The listing builds one solid part. Answer for the finished solid, in the listing's coordinates (mm). Coordinates: 2 decimals unless noted, no trailing zeros. Write each loop counter-clockwise with the first axis right and the second up, starting at its lowest first coordinate (ties: lowest second). Pieces come first, ordered by that corner, then holes. Notation, with made-up numbers: M 62,-19 L 93,-19 A24 ccw 93,-9 Z; hole C 44,19.5 d1. An arc over 180 degrees is marked long. Answer as CSV lines item,"result".
```python
from build123d import *

# Parameters (mm, degrees)
SKETCH_1_R      = 3.127436884
SKETCH_1_R_2    = 2.290236854
SKETCH_1_R_3    = 3.334332824
SKETCH_1_R_4    = 3
SKETCH_1_R_5    = 1.883976709
SKETCH_1_R_6    = 2.353930843
SKETCH_1_R_7    = 1.55
EXTRUDE_1_DEPTH = 1.5


with BuildPart() as part:
    # 草图1 → 凸台-拉伸1 (new body)
    with BuildSketch(Plane(origin=(0, 0, 0), x_dir=(1, 0, 0), z_dir=(0, 1, 0))):
        Polygon((-30, 10), (-30, 0), (0, 0), (30, 0), (30, 10), align=None)
        with Locations((17.823374051, 5.840236854)):
            Circle(SKETCH_1_R, mode=Mode.SUBTRACT)
        with Locations((12.171443923, 3.55)):
            Circle(SKETCH_1_R_2, mode=Mode.SUBTRACT)
        with Locations((4.963185209, 5.738422027)):
            Circle(SKETCH_1_R_3, mode=Mode.SUBTRACT)
        with Locations((-4.210962245, 6.229894212)):
            Circle(SKETCH_1_R_4, mode=Mode.SUBTRACT)
        with Locations((-12.074517206, 2.707676886)):
            Circle(SKETCH_1_R_5, mode=Mode.SUBTRACT)
        with Locations((-17.808359365, 7)):
            Circle(SKETCH_1_R_6, mode=Mode.SUBTRACT)
        with Locations((-26.9, 2)):
            Circle(SKETCH_1_R_7, mode=Mode.SUBTRACT)
        with Locations((-26.9, 7)):
            Circle(SKETCH_1_R_7, mode=Mode.SUBTRACT)
        with Locations((26.9, 7)):
            Circle(SKETCH_1_R_7, mode=Mode.SUBTRACT)
        with Locations((26.9, 2)):
            Circle(SKETCH_1_R_7, mode=Mode.SUBTRACT)
    extrude(amount=EXTRUDE_1_DEPTH)


solid = part.part
```
Q1. Find section B-B (z = -7). Give the vertices of the cut face in (x, y).
Output:
outline,"M -30,0 L -28.45,0 L -28.45,1.5 L -30,1.5 Z; M -25.35,0 L -20.16,0 L -20.16,1.5 L -25.35,1.5 Z; M -15.45,0 L -7.11,0 L -7.11,1.5 L -15.45,1.5 Z; M -1.31,0 L 1.88,0 L 1.88,1.5 L -1.31,1.5 Z; M 8.05,0 L 14.92,0 L 14.92,1.5 L 8.05,1.5 Z; M 20.73,0 L 25.35,0 L 25.35,1.5 L 20.73,1.5 Z; M 28.45,0 L 30,0 L 30,1.5 L 28.45,1.5 Z"
Q2. The mould has two halves that part along X. Classify faces 1 (the cylindrical face through (28.332, 0.74, -6.406)), 2 (the flat face through (-30, 1, -5)), 3 (the flat face through (0, 1, -10)): pulls with the +X half, pulls with the -X half, needs draft (parallel to the pull), parting line crosses it, or undercut.
Output:
face 1,"undercut"
face 2,"pulls with the -X half"
face 3,"needs draft"
Q3. Find section D-D (y = 1). Count the separate pieces of the cut face and the enclosed holes in it, and give its area (3 significant figures).
Output:
separate pieces,"1"
enclosed holes,"10"
area,"431 mm2"
Q4. Find section C-C (x = 13.5). Give the vertices of the cut face in (y, z).
Output:
outline,"M 0,-10 L 1.5,-10 L 1.5,-5.42 L 0,-5.42 Z; M 0,-1.68 L 1.5,-1.68 L 1.5,0 L 0,0 Z"
Q5. Straight lines are drawn through the part: line 1 (Z direction, x = -26.9, y = 0.4); line 2 (X direction, y = 0.5, z = -1.5); line 3 (X direction, y = 0.8, z = -2.25). For each, find the intervals that lie inside material, in ascending order.
Output:
line 1,"-10 to -8.55, -5.45 to -3.55, -0.45 to 0"
line 2,"-30 to -28.37, -25.43 to -13.52, -10.63 to 11.15, 13.19 to 25.43, 28.37 to 30"
line 3,"-30 to -28.43, -25.37 to -13.9, -10.25 to 10.29, 14.06 to 25.37, 28.43 to 30"
Q6. Find section A-A (x = 26.9). Give the vertices of the cut face in (y, z), and give its area (3 significant figures).
Output:
outline,"M 0,-10 L 1.5,-10 L 1.5,-8.55 L 0,-8.55 Z; M 0,-5.45 L 1.5,-5.45 L 1.5,-3.55 L 0,-3.55 Z; M 0,-0.45 L 1.5,-0.45 L 1.5,0 L 0,0 Z"
area,"5.70 mm2"
